Autodesk Inventor part; units mm, degrees
ref_plane "YZ Plane" through (0, 0, 0) normal (1, 0, 0) x (0, 1, 0)
ref_plane "XZ Plane" through (0, 0, 0) normal (0, 1, 0) x (-1, 0, 0)
ref_plane "XY Plane" through (0, 0, 0) normal (0, 0, 1) x (1, 0, 0)
sketch "Sketch1" plane through (0, 0, 0) normal (0, 0, 1) x (1, 0, 0)
  circle A0 centre (0, 0) radius 3
  dimension "d0" = 6
extrude "Extrusion1" add sketch "Sketch1" along normal mid plane 25
sketch "Sketch2" plane through (0, 0, 12.5) normal (0, 0, 1) x (1, 0, 0)
  point P0 (0, 0)
  point P1 (2.8235, 0.7984)
hole "Hole1" at (0, 0, 12.5) direction (0, 0, -1) diameter 3.242 end up to surface
chamfer "Chamfer1" distance 0.25 angle 45 2 edges at (-3, 0, 12.5) (-3, 0, -12.5)
properties part number "FootPin" material "Acetal Resin, White"
Check sheet for the modelled part. Datum: model origin and axes. Units: mm. Give positions to 0.01 mm unless a question says otherwise; leave off trailing zeros. Write each loop counter-clockwise with the first axis right and the second up, starting at its lowest first coordinate (ties: lowest second). Pieces come first, ordered by that corner, then holes. Notation, with made-up numbers: (43, 45) -> (62, 45) arc R4 ccw to (62, 49) -> close; hole circle Ø6 at (35, 84.25). An arc over 180 degrees is marked (long way). One line per item, written item: value. Start each with the question number.
Item 1: Gauge pin test, flat end, axial feed: pin 1 (1.5 mm diameter, centred on x = -1.5, z = -2, fed in from +Y). Record the tip position at first contact, or that the pin passes through.
Item 2: Section check A-A on y = 0. Record the cut outline in (x, z).
Item 3: Section check B-B on z = -4.25. Record the cut outline in (x, y), then the cut area to 3 significant figures.
Item 4: Draft check along X on faces 1 (the cylindrical face through (-3, 0, 0)), 2 (the flat face through (2, 0, -12.5)), 3 (the cylindrical face through (1.438, -0.748, -0.175)). Enter one of: +X half, -X half, draft (parallel to the pull), parting line (faces both ways), or undercut.
Item 5: Material ranges on probe 1 along Y at (x, z) = (0.05, -0.75); probe 2 along X at (y, z) = (-1.3, -10.5), recorded low to high. Write a range as from..to.
Results list:
1. pin 1: y = 2.9
2. outline: (-3, -12.25) -> (-2.75, -12.5) -> (-1.62, -12.5) -> (-1.62, 12.5) -> (-2.75, 12.5) -> (-3, 12.25) -> close; (1.62, -12.5) -> (2.75, -12.5) -> (3, -12.25) -> (3, 12.25) -> (2.75, 12.5) -> (1.62, 12.5) -> close
3. outline: circle Ø6 at (0, 0); hole circle Ø3.24 at (0, 0)
3. area: 20.0 mm²
4. face 1: parting line
4. face 2: draft
4. face 3: undercut
5. probe 1: -3..-1.62, 1.62..3
5. probe 2: -2.7..-0.97, 0.97..2.7
